Autodesk Inventor part; units mm, degrees
ref_plane "YZ Plane" through (0, 0, 0) normal (1, 0, 0) x (0, 1, 0)
ref_plane "XZ Plane" through (0, 0, 0) normal (0, 1, 0) x (-1, 0, 0)
ref_plane "XY Plane" through (0, 0, 0) normal (0, 0, 1) x (1, 0, 0)
sketch "スケッチ1" plane through (0, 0, 0) normal (0, 0, 1) x (1, 0, 0)
  line L0 (0, 49.5) -> (30, 49.5)
  line L1 (0, 0) -> (30, 0)
  line L2 (0, 0) -> (0, 49.5)
  line L3 (30, 0) -> (30, 49.5)
  dimension "d2" = 30
  dimension "d38" = 49.5
extrude "押し出し1" add sketch "スケッチ1" along normal blind 5
sketch "スケッチ4" plane through (30, 0, 0) normal (1, 0, 0) x (0, 0, -1)
  line L0 (0, 49.5) -> (-5, 49.5)
  line L1 (-2.5, 49.5) -> (-2.5, 0) construction
  line L2 (0, 0) -> (-5, 0)
  point P0 (0, 0)
  point P1 (-2.5, 47)
  point P2 (-2.5, 2.5)
  point P3 (-2.5, 7.5)
  point P4 (-2.5, 12.5)
  dimension "d22" = 2.5
  dimension "d40" = 2.5
  dimension "d41" = 5
  dimension "d42" = 5
hole "穴1" at (30, 47, 2.5) direction (-1, 0, 0) diameter 3.1 depth 5
sketch "スケッチ5" plane through (0, 0, 0) normal (-1, 0, 0) x (0, 0, 1)
  circle A0 centre (2.5, 47) radius 1.55
  line L0 (0, 0) -> (5, 0)
  line L1 (2.5, 0) -> (2.5, 49.5) construction
  line L2 (0, 49.5) -> (5, 49.5)
  point P0 (2.5, 2.5)
  point P1 (2.5, 7.5)
  point P2 (2.5, 12.5)
  dimension "d50" = 2.5
  dimension "d51" = 5
  dimension "d52" = 5
hole "穴2" at (0, 47, 2.5) direction (1, 0, 0) diameter 3.1 depth 5
hole "穴5" at (30, 2.5, 2.5) at (30, 12.5, 2.5) at (30, 7.5, 2.5) direction (-1, 0, 0) diameter 3 depth 3
hole "穴6" at (0, 2.5, 2.5) at (0, 7.5, 2.5) at (0, 12.5, 2.5) direction (1, 0, 0) diameter 3 depth 3
properties part number "Cockpit_vertical_frame_07" material "アセタール樹脂、黒"
Source: CAD feature listing. Evaluate the final solid. Frame: model axes, mm. A direction names the side the tool comes from. Give positions to 0.01 mm unless a question says otherwise; leave off trailing zeros. Loops run counter-clockwise (first coordinate to the right, second up) from the corner with the lowest first, then second, coordinate; pieces in that order, holes last. Notation, with made-up numbers: (-1.75, 18.25) -> (50.25, 18.25) arc R25 cw to (50.25, 40.25) -> close; hole circle Ø5 at (17.25, 73). An arc over 180 degrees is marked (long way). Use a Markdown table: item, result. Add a question column.
1) First-contact query: pin 1 (2.5 mm diameter, centred on y = 12.5, z = 2.5, fed in from +X); pin 2 (1.8 mm diameter, centred on y = 2.5, z = 2.5, fed in from -X); pin 3 (2.5 mm diameter, centred on y = 47, z = 2.5, fed in from -X). Flat tips, straight axial feed; report the tip coordinate or a pass-through.
2) Pull-direction query (Z, two-part tool) for faces 4 (the face through (0, 24, 2)), 5 (the face through (15, 25, 5)), 6 (the face through (28.479, 8.964, 2.825)); classes: +Z half, -Z half, draft (parallel to the pull), parting line (faces both ways), or undercut.
3) Line query: line 1 along Y through (x, z) = (1.75, 2.5); line 2 along Z through (x, y) = (28.35, 12.5); line 3 along Y through (x, z) = (2.75, 3.4). Output: solid intervals per line, ascending. Write a range as [from, to].
4) Section query A-A, the plane y = 47. Return the cut outline in (x, z), then the cut area to 3 significant figures.
5) Reachability of faces 1 (the face through (30, 24, 2)), 2 (the face through (27.465, 48.513, 2.836)), 3 (the face through (2.535, 48.513, 2.164)) from +Z, -Z, +X, -X, +Y, -Y: full face, straight path, thin tool, end or side. Return the list, or none.
6) Section query B-B, the plane y = 7.5. Return the cut outline in (x, z), then the cut area to 3 significant figures.
Numbers:
| question | item | result |
|---|---|---|
| 1 | pin 1 | stops at x = 27 |
| 1 | pin 2 | stops at x = 3 |
| 1 | pin 3 | stops at x = 5 |
| 2 | face 4 | draft |
| 2 | face 5 | +Z half |
| 2 | face 6 | undercut |
| 3 | line 1 | y = [0, 1], [4, 6], [9, 11], [14, 45.45], [48.55, 49.5] |
| 3 | line 2 | z = [0, 1], [4, 5] |
| 3 | line 3 | y = [0, 1.3], [3.7, 6.3], [8.7, 11.3], [13.7, 45.74], [48.26, 49.5] |
| 4 | outline | (0, 0) -> (30, 0) -> (30, 0.95) -> (25, 0.95) -> (25, 4.05) -> (30, 4.05) -> (30, 5) -> (0, 5) -> (0, 4.05) -> (5, 4.05) -> (5, 0.95) -> (0, 0.95) -> close |
| 4 | area | 119 mm2 |
| 5 | face 1 | +Z, -Z, +X, +Y, -Y |
| 5 | face 2 | +X |
| 5 | face 3 | -X |
| 6 | outline | (0, 0) -> (30, 0) -> (30, 1) -> (27, 1) -> (27, 4) -> (30, 4) -> (30, 5) -> (0, 5) -> (0, 4) -> (3, 4) -> (3, 1) -> (0, 1) -> close |
| 6 | area | 132 mm2 |
